Geometry check sheet. Reference: the model listing, model coordinates, mm. Face numbers are marked on the shaded views. A direction names the side the tool comes from. Round coordinates to 2 decimals unless told otherwise and drop trailing zeros. Order: outer loops, then holes, each group sorted by start corner. A loop starts at its lowest first (then second) coordinate and runs counter-clockwise, first axis right, second up.
(1) Sectioned sample at A-A (y = 8.25). Record the boundary of the cut face in (x, z).
(2) Set-up check for the marked faces 1, 2 and 3: record each of +Z, -Z, +X, -X, +Y, -Y from which the full face is reachable in a straight line by a thin tool's end or side.
(3) Go/stop test with flat-tipped pins: pin 1 (1.3 mm diameter, centred on x = -0.5, y = 11.5, fed in from -Z); pin 2 (1 mm diameter, centred on x = -2.5, z = -3, fed in from -Y); pin 3 (5 mm diameter, centred on y = 6.5, z = -3, fed in from -X); pin 4 (5 mm diameter, centred on x = 0.5, z = -3, fed in from -Y). Record where each tip stops, or that it passes through.
(4) Material ranges on line 1 along Y through (x, z) = (0.5, 0.5); line 2 along Y through (x, z) = (2, -0.5); line 3 along Z through (x, y) = (0, 5.5), recorded low to high.
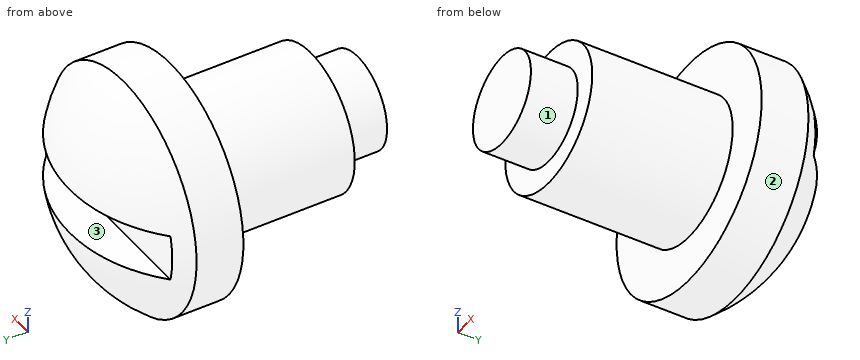
from build123d import *

# Parameters (mm, degrees)
KES_EKSTR_ZYON12_START = -4.399452
IZIM9_W                = 2
IZIM9_H                = 1.732554961
KES_EKSTR_ZYON12_DEPTH = 8.798904


with BuildPart() as part:
    # Çizim2 → Döndür3 (revolve)
    with BuildSketch(Plane.XY):
        with BuildLine():
            Line((0, 0), (2, 0))
            Line((2, 0), (2, 2))
            Line((2, 2), (3, 2))
            Line((3, 2), (3, 8))
            Line((3, 8), (5, 8))
            Line((5, 8), (5, 10))
            ThreePointArc((5, 10), (2.783322768, 11.790255766), (0, 12.4))
            Line((0, 12.4), (0, 0))
        make_face()
    revolve(axis=Axis((0, 0, 0), (0, 1, 0)))

    # Çizim9 → Kes-Ekstrüzyon12 (cut)
    with BuildSketch(Plane(origin=(0, 0, 0), x_dir=(0, 0, -1), z_dir=(1, 0, 0)).offset(KES_EKSTR_ZYON12_START)):
        with Locations((0, 11.53453533)):
            Rectangle(IZIM9_W, IZIM9_H)
    kes_ekstr_zyon12 = extrude(amount=KES_EKSTR_ZYON12_DEPTH, mode=Mode.SUBTRACT)

    # Aynalama2: Kes-Ekstrüzyon12 across plane
    add(kes_ekstr_zyon12.mirror(Plane(origin=(0, 0, 0), x_dir=(0, 0, 1), z_dir=(1, 0, 0))), mode=Mode.SUBTRACT)


solid = part.part
Answer below:
1. outline: circle Ø10 at (0, 0)
2. face 1: -Y
2. face 2: +Y, -Y
2. face 3: +X, -X, +Y
3. pin 1: stops at z = -4.18
3. pin 2: stops at y = 8
3. pin 3: stops at x = -4.9
3. pin 4: stops at y = 0
4. line 1: y = 0 to 10.67
4. line 2: y = 2 to 10.67
4. line 3: z = -3 to 3
